The figure shows three views and two pictorial views of one solid part (mm, origin at its lowest corner). Answer the questions. A direction names the side the tool comes from. Coordinates: 2 decimals unless noted, no trailing zeros. Order: outer loops, then holes, each group sorted by start corner. A loop starts at its lowest first (then second) coordinate and runs counter-clockwise, first axis right, second up. Notation, with made-up numbers: (-32, 31.25) - (-4, 31.25) arc R9 cw to (-4, 48.25) - close; hole circle Ø10 at (37.25, -30.5). An arc over 180 degrees is marked (long way). Use one line per item in the form item = value. Start each with the question number.
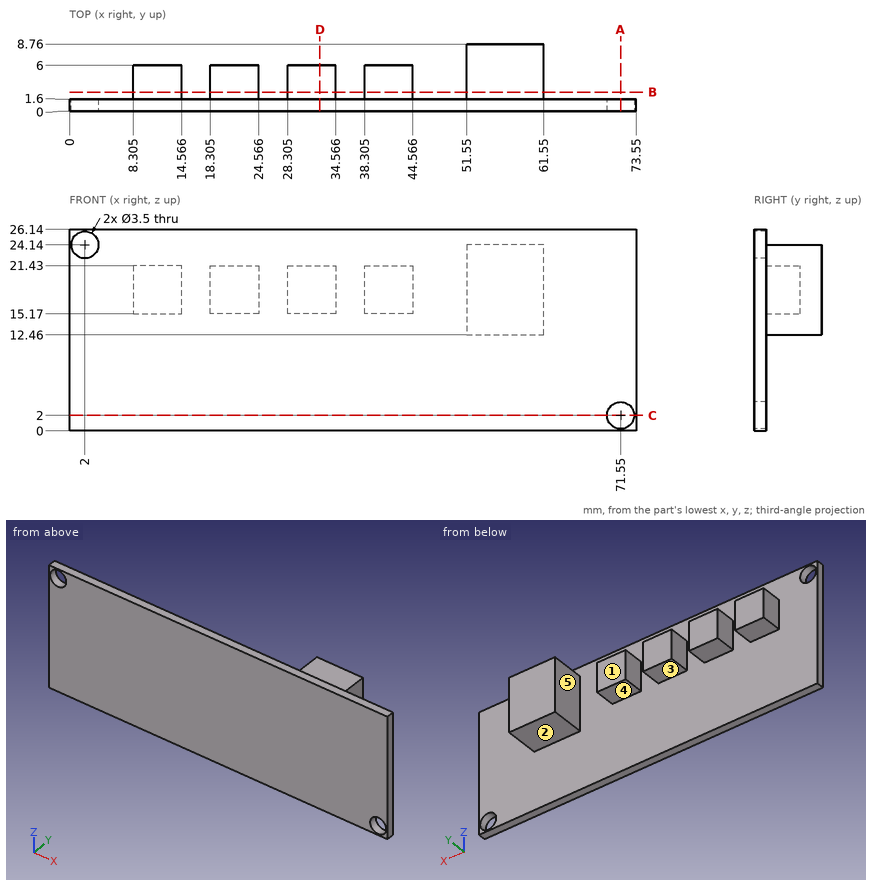
Q1. Consider probe 1 along Z at (x, y) = (71.55, 0.7); probe 2 along Y at (x, z) = (19.5, 18.5); probe 3 along Y at (x, z) = (62, 21.5). Determine where each line is inside the solid, lowest interval first.
Q2. Which of the six approach directions +Z, -Z, +X, -X, +Y, -Y give full straight-line access (tool end or side, diameter ignored) to the marked faces 1, 2 and 3?
Q3. For a pull along X with two mould halves and no side action, classify the marked faces 4 and 5 as +X half, -X half, draft (parallel to the pull), parting line (faces both ways), or undercut.
Q4. A cutting plane is placed at D-D (x = 32.5). Give the vertices of the cut face in (y, z).
Q5. A cutting plane is placed at C-C (z = 2). Give the vertices of the cut face in (x, y).
Q6. A cutting plane is placed at B-B (y = 2.5). Give the number of separate pieces and of enclosed holes in the cut face.
Q7. Given P1, Ø2, axis at y = 6, z = 19, coming from the +X side; P2, Ø2, axis at x = 20.5, y = 3.5, coming from the +Z side; P3, Ø10, axis at x = 66, z = 3, coming from the -Y side; P4, Ø3, axis at y = 4.5, z = 20, coming from the -X side (1 decimal), each flat-ended and moving along its own axis, determine where each tip first touches the part or whether it passes through.
Q8. A cutting plane is placed at A-A (x = 71.55). Give the vertices of the cut face in (y, z).
Result sheet:
q1.probe_1 = 0 to 0.25, 3.75 to 26.14
q1.probe_2 = 0 to 6
q1.probe_3 = 0 to 1.6
q2.face_1 = +Z, -Z, -X, +Y
q2.face_2 = -Z, +X, -X, +Y
q2.face_3 = -Z, -X, +Y
q3.face_4 = draft
q3.face_5 = undercut
q4.outline = (0, 0) - (1.6, 0) - (1.6, 15.17) - (6, 15.17) - (6, 21.43) - (1.6, 21.43) - (1.6, 26.14) - (0, 26.14) - close
q5.outline = (0, 0) - (69.8, 0) - (69.8, 1.6) - (0, 1.6) - close; (73.3, 0) - (73.55, 0) - (73.55, 1.6) - (73.3, 1.6) - close
q6.separate_pieces = 5
q6.enclosed_holes = 0
q7.P1 = 61.55
q7.P2 = 21.43
q7.P3 = 0
q7.P4 = 8.3
q8.outline = (0, 0) - (1.6, 0) - (1.6, 0.25) - (0, 0.25) - close; (0, 3.75) - (1.6, 3.75) - (1.6, 26.14) - (0, 26.14) - close
